CAD build for the part. Positions are in the model's coordinates, mm. A direction names the side the tool comes from. Give positions to 0.01 mm unless a question says otherwise; leave off trailing zeros. Write each loop counter-clockwise with the first axis right and the second up, starting at its lowest first coordinate (ties: lowest second). Pieces come first, ordered by that corner, then holes. Notation, with made-up numbers: (70.25, 49) - (119.25, 49) arc R21 cw to (119.25, 68) - close; hole circle Ø11 at (23.25, 20). An arc over 180 degrees is marked (long way). Answer as a JSON object with one key per item and string values.
from build123d import *

# Parameters (mm, degrees)
F1_R     = 8
F3_T     = -1.5
F5_D     = 10
F5_DEPTH = 318.0010001
F6_D     = 10


with BuildPart() as f2:
    # F2: sweep along a path in F0
    with BuildLine(Plane.YZ) as f2_path:
        Line((-310, 0), (-310, 750))
        ThreePointArc((-310, 750), (-280.7106781187, 820.7106781187), (-210, 850))
        Line((-210, 850), (-100, 850))
        ThreePointArc((-100, 850), (-29.2893218813, 820.7106781187), (0, 750))
        Line((0, 750), (0, 0))
    # F1 (on Top) → F2 (sweep)
    with BuildSketch(Plane.XY):
        Circle(F1_R)
    sweep(path=f2_path.line)

    # F3
    f3_openings = [f2.faces().sort_by_distance(p)[0] for p in [
        (0, -310, 0),
        (0, 0, 0),
    ]]
    offset(amount=F3_T, openings=f3_openings)

    # F5 (through all, one way)
    with BuildSketch(Plane(origin=(0, 0, 0), x_dir=(1, 0, 0), z_dir=(0, 1, 0))):
        with Locations((0, -425)):
            Circle(F5_D / 2)
    extrude(amount=-F5_DEPTH, mode=Mode.SUBTRACT)

    # F6 (through all)
    with Locations(Plane.XZ):
        with Locations((0, 425)):
            Hole(F6_D / 2)


solid = f2.part
(1) 3-axis set-ups, long thin cutter, end or side, ignore diameter. For faces 1 (the face through (3.69, -154.23, 857.1)), 2 (the face through (0, 7, 0)): which of +Z, -Z, +X, -X, +Y, -Y reach the whole face in a straight line?
Answer key:
{"face 1": "none", "face 2": "-Z, +X, -X, +Y, -Y"}
(2) Saw through at A-A, the plane z = 117.5. Give the cut face in (x, y).
Answer key:
{"outline": "circle Ø16 at (0, -310); circle Ø16 at (0, 0); hole circle Ø13 at (0, -310); hole circle Ø13 at (0, 0)"}
(3) Pull direction Y, two halves, no side cores. Call faces 3 (the face through (0, -303, 0)), 4 (the face through (-1.041, -302.068, 380.25)), 5 (the face through (-1.73, 7.81, 369.75)): pulls with the +Y half, pulls with the -Y half, needs draft (parallel to the pull), parting line crosses it, or undercut.
Answer key:
{"face 3": "needs draft", "face 4": "undercut", "face 5": "undercut"}
(4) Saw through at B-B, the plane y = -196. Give the cut face in (x, z).
Answer key:
{"outline": "circle Ø16 at (0, 850); hole circle Ø13 at (0, 850)"}
(5) Saw through at C-C, the plane x = 0. State how many separate pieces and enclosed holes the cut face has, and give its area (3 significant figures).
Answer key:
{"separate pieces": "6", "enclosed holes": "0", "area": "5,710 mm²"}
(6) Flat gauge pins, fed straight in: P1, Ø5, axis at x = 4.5, y = -86, coming from the +Z side; P2, Ø3, axis at x = 6.5, y = -128, coming from the +Z side (3 decimals); P3, Ø2, axis at x = 1.5, z = 305.5, coming from the -Y side. Where does each tip first touch, or does it go through?
Answer key:
{"P1": "stops at z = 856.9", "P2": "stops at z = 856.245", "P3": "stops at y = -317.98"}
(7) Probe L1, parallel to Y at x = 0, z = 199.5; L2, parallel to X at y = -158, z = 850; L3, parallel to Y at x = -1, z = 740. List the from-to ranges inside material, lowest first. Write a range as [from, to].
Answer key:
{"L1": "y = [-318, -316.5], [-303.5, -302], [-8, -6.5], [6.5, 8]", "L2": "x = [-8, -6.5], [6.5, 8]", "L3": "y = [-317.94, -316.42], [-303.58, -302.06], [-7.94, -6.42], [6.42, 7.94]"}
